Verification items for the finished model (mm, model axes). A direction names the side the tool comes from. Round coordinates to 2 decimals unless told otherwise and drop trailing zeros. Order: outer loops, then holes, each group sorted by start corner. A loop starts at its lowest first (then second) coordinate and runs counter-clockwise, first axis right, second up. Notation, with made-up numbers: (5, 61) -> (46, 61) arc R9 cw to (46, 74) -> close; hole circle Ø4 at (59.5, -17). An arc over 180 degrees is marked (long way). Return JSON: item names as keys, results as strings. Group by question number.
1) Tool access check on faces 4 (the flat face through (61.7, 2, 1)), 5 (the flat face through (20, 6.426, 1)), 6 (the flat face through (54.8, -17, 1)), 7 (the flat face through (61, 13.92, 1)). Record the directions out of +Z, -Z, +X, -X, +Y, -Y that give a thin tool (end or side, any length) a straight path to the whole face; none if there is none.
2) Section check C-C on y = 3. Enter the section's corners in (x, z), plus the area to 3 significant figures.
3) Scan lines: L1, parallel to Y at x = 63.3, z = 1.45; L2, parallel to Y at x = 19.5, z = 0.65; L3, parallel to X at y = 0, z = 0.5. Record each from-to range of solid material in increasing order.
4) Depth check by flat-ended pin: pin 1 (1.5 mm diameter, centred on x = 61.5, z = 1.5, fed in from -Y); pin 2 (1.5 mm diameter, centred on y = 2, z = 1, fed in from -X); pin 3 (1.6 mm diameter, centred on x = 15.5, z = 1.5, fed in from -Y); pin 4 (12 mm diameter, centred on x = 59, y = -8.5, fed in from -Z). Enter the tip coordinate at first touch or a pass-through.
5) Section check A-A on x = 19.5. Enter the section's corners in (y, z).
6) Draft check along Y on faces 1 (the flat face through (39.8, -17, 1)), 2 (the flat face through (31, -15.18, 1)), 3 (the flat face through (38.14, 2.58, 1.48)). Enter one of: pulls with the +Y half, pulls with the -Y half, needs draft (parallel to the pull), parting line crosses it, or undercut.
7) Section check B-B on x = 62.5. Enter the section's corners in (y, z).
8) Section check D-D on z = 1.65. State how many separate pieces and enclosed holes the cut face has, plus the area to 3 significant figures.
```python
from build123d import *

# Parameters (mm, degrees)
SKETCH_1_R           = 1.8
SKETCH_1_W           = 3
SKETCH_1_H           = 12
EXTRUDE_1_DEPTH      = 3
SKETCH_3_W           = 34
SKETCH_3_H           = 3
CUT_EXTRUDE_1_DEPTH  = 10
SKETCH_4_W           = 38
SKETCH_4_H           = 2
CUT_EXTRUDE_2_DEPTH  = 10
SKETCH_5_W           = 3
SKETCH_5_H           = 2
EXTRUDE_2_DEPTH      = 2
SKETCH_6_W           = 3
SKETCH_6_H           = 2
EXTRUDE_3_DEPTH      = 2
SKETCH_7_W           = 34
SKETCH_7_H           = 3
CUT_EXTRUDE_3_DEPTH  = 2
SKETCH_8_W           = 3
SKETCH_8_H           = 10
EXTRUDE_4_DEPTH      = 5
SKETCH_9_W           = 5
SKETCH_9_H           = 3
CUT_EXTRUDE_4_DEPTH  = 2
CUT_EXTRUDE_5_DEPTH  = 10
SKETCH_11_W          = 3
SKETCH_11_H          = 8
CUT_EXTRUDE_6_DEPTH  = 5
SKETCH_12_W          = 3.2
SKETCH_12_H          = 12.2
SKETCH_12_W_2        = 3
SKETCH_12_H_2        = 12
CUT_EXTRUDE_7_DEPTH  = 10
SKETCH_13_W          = 3.2
SKETCH_13_H          = 3
EXTRUDE_5_DEPTH      = 3
SKETCH_14_W          = 3.2
SKETCH_14_H          = 3
CUT_EXTRUDE_8_DEPTH  = 3
SKETCH_15_W          = 3.2
SKETCH_15_H          = 3
EXTRUDE_6_DEPTH      = 1
SKETCH_16_R          = 1.4
CUT_EXTRUDE_9_DEPTH  = 3
SKETCH_17_W          = 5
SKETCH_17_H          = 3.106186253
CUT_EXTRUDE_10_DEPTH = 10


with BuildPart() as part:
    # 草图1 → 凸台-拉伸1 (new body)
    with BuildSketch(Plane.XY):
        Polygon((-64.8, 13.92), (-67.8, 13.92), (-70.8, 10.92), (-70.8, -12.18), (-67.8, -15.18), (-64.8, -15.18), (-54.8, -15.18), (-54.8, -17.98), (-39.8, -17.98), (-39.8, -15.18), (-22, -15.18), (-22, 3.32), (-17, 3.32), (-17, 0.32), (17, 0.32), (17, 3.32), (22, 3.32), (22, -15.18), (39.8, -15.18), (39.8, -17.98), (54.8, -17.98), (54.8, -15.18), (67.8, -15.18), (70.8, -12.18), (70.8, 10.92), (67.8, 13.92), (54.8, 13.92), (54.8, 16.72), (29.8, 16.72), (29.8, 13.92), (10, 13.92), (10, 16.72), (-10, 16.72), (-10, 13.92), (-29.8, 13.92), (-29.8, 16.72), (-54.8, 16.72), (-54.8, 13.92), align=None)
        with Locations((-19.5, 10.636938849)):
            Circle(SKETCH_1_R, mode=Mode.SUBTRACT)
        with Locations((19.5, 10.636938849)):
            Circle(SKETCH_1_R, mode=Mode.SUBTRACT)
        with BuildLine():
            Line((-48.112743691, -4.863700543), (-43.239089288, 0.009953861))
            ThreePointArc((-43.239089288, 0.009953861), (-43.026957254, 0.097821826), (-42.814825219, 0.009953861))
            Line((-42.814825219, 0.009953861), (-40.739089288, -2.065782071))
            ThreePointArc((-40.739089288, -2.065782071), (-40.651221322, -2.277914105), (-40.739089288, -2.490046139))
            Line((-40.739089288, -2.490046139), (-43.380510644, -5.131467496))
            ThreePointArc((-43.380510644, -5.131467496), (-44.029357342, -5.565012998), (-44.794724207, -5.717253933))
            Line((-44.794724207, -5.717253933), (-47.759190301, -5.717253933))
            ThreePointArc((-47.759190301, -5.717253933), (-48.221130067, -5.408595649), (-48.112743691, -4.863700543))
        make_face(mode=Mode.SUBTRACT)
        with Locations((-63.3, -0.08)):
            Rectangle(SKETCH_1_W, SKETCH_1_H, mode=Mode.SUBTRACT)
        with BuildLine():
            Line((-37.309442832, -3.374108183), (-45.06249116, 4.378940145))
            ThreePointArc((-45.06249116, 4.378940145), (-45.170877535, 4.923835251), (-44.708937769, 5.232493535))
            Line((-44.708937769, 5.232493535), (-43.744471675, 5.232493535))
            ThreePointArc((-43.744471675, 5.232493535), (-42.97910481, 5.0802526), (-42.330258113, 4.646707097))
            Line((-42.330258113, 4.646707097), (-34.577209785, -3.10634123))
            ThreePointArc((-34.577209785, -3.10634123), (-34.46882341, -3.651236336), (-34.930763176, -3.95989462))
            Line((-34.930763176, -3.95989462), (-35.89522927, -3.95989462))
            ThreePointArc((-35.89522927, -3.95989462), (-36.660596135, -3.807653685), (-37.309442832, -3.374108183))
        make_face(mode=Mode.SUBTRACT)
        with BuildLine():
            Line((-32.819850472, 5.429192676), (-36.693504876, 1.555538273))
            ThreePointArc((-36.693504876, 1.555538273), (-36.90563691, 1.467670307), (-37.117768944, 1.555538273))
            Line((-37.117768944, 1.555538273), (-39.193504876, 3.631274204))
            ThreePointArc((-39.193504876, 3.631274204), (-39.281372841, 3.843406239), (-39.193504876, 4.055538273))
            Line((-39.193504876, 4.055538273), (-37.55208352, 5.696959629))
            ThreePointArc((-37.55208352, 5.696959629), (-36.903236822, 6.130505132), (-36.137869957, 6.282746067))
            Line((-36.137869957, 6.282746067), (-33.173403863, 6.282746067))
            ThreePointArc((-33.173403863, 6.282746067), (-32.711464097, 5.974087783), (-32.819850472, 5.429192676))
        make_face(mode=Mode.SUBTRACT)
        with Locations((63.3, -0.076886306)):
            Rectangle(SKETCH_1_W, SKETCH_1_H, mode=Mode.SUBTRACT)
        with BuildLine():
            Line((42.330258113, 4.646707097), (34.577209785, -3.10634123))
            ThreePointArc((34.577209785, -3.10634123), (34.46882341, -3.651236336), (34.930763176, -3.95989462))
            Line((34.930763176, -3.95989462), (35.89522927, -3.95989462))
            ThreePointArc((35.89522927, -3.95989462), (36.660596135, -3.807653685), (37.309442832, -3.374108183))
            Line((37.309442832, -3.374108183), (45.06249116, 4.378940145))
            ThreePointArc((45.06249116, 4.378940145), (45.170877535, 4.923835251), (44.708937769, 5.232493535))
            Line((44.708937769, 5.232493535), (43.744471675, 5.232493535))
            ThreePointArc((43.744471675, 5.232493535), (42.97910481, 5.0802526), (42.330258113, 4.646707097))
        make_face(mode=Mode.SUBTRACT)
        with BuildLine():
            Line((48.112743691, -4.863700543), (43.239089288, 0.009953861))
            ThreePointArc((43.239089288, 0.009953861), (43.026957254, 0.097821826), (42.814825219, 0.009953861))
            Line((42.814825219, 0.009953861), (40.739089288, -2.065782071))
            ThreePointArc((40.739089288, -2.065782071), (40.651221322, -2.277914105), (40.739089288, -2.490046139))
            Line((40.739089288, -2.490046139), (43.380510644, -5.131467496))
            ThreePointArc((43.380510644, -5.131467496), (44.029357342, -5.565012998), (44.794724207, -5.717253933))
            Line((44.794724207, -5.717253933), (47.759190301, -5.717253933))
            ThreePointArc((47.759190301, -5.717253933), (48.221130067, -5.408595649), (48.112743691, -4.863700543))
        make_face(mode=Mode.SUBTRACT)
        with BuildLine():
            Line((39.193504876, 4.055538273), (37.55208352, 5.696959629))
            ThreePointArc((37.55208352, 5.696959629), (36.903236822, 6.130505132), (36.137869957, 6.282746067))
            Line((36.137869957, 6.282746067), (33.173403863, 6.282746067))
            ThreePointArc((33.173403863, 6.282746067), (32.711464097, 5.974087783), (32.819850472, 5.429192676))
            Line((32.819850472, 5.429192676), (36.693504876, 1.555538273))
            ThreePointArc((36.693504876, 1.555538273), (36.90563691, 1.467670307), (37.117768944, 1.555538273))
            Line((37.117768944, 1.555538273), (39.193504876, 3.631274204))
            ThreePointArc((39.193504876, 3.631274204), (39.281372841, 3.843406239), (39.193504876, 4.055538273))
        make_face(mode=Mode.SUBTRACT)
    extrude(amount=EXTRUDE_1_DEPTH)

    # 草图3 → 切除-拉伸1 (cut)
    with BuildSketch(Plane(origin=(0, 0, 0), x_dir=(-1, 0, 0), z_dir=(0, 0, -1))):
        with Locations((0, 1.82)):
            Rectangle(SKETCH_3_W, SKETCH_3_H)
    extrude(amount=-CUT_EXTRUDE_1_DEPTH, mode=Mode.SUBTRACT)

    # 草图4 → 切除-拉伸2 (cut)
    with BuildSketch(Plane(origin=(0, 0, 0), x_dir=(-1, 0, 0), z_dir=(0, 0, -1))):
        with Locations((0, 4.32)):
            Rectangle(SKETCH_4_W, SKETCH_4_H)
    extrude(amount=-CUT_EXTRUDE_2_DEPTH, mode=Mode.SUBTRACT)

    # 草图5 → 凸台-拉伸2 (add)
    with BuildSketch(Plane(origin=(-19, 0, 0), x_dir=(0, 0, -1), z_dir=(1, 0, 0))):
        with Locations((-1.5, 4.32)):
            Rectangle(SKETCH_5_W, SKETCH_5_H)
    extrude(amount=EXTRUDE_2_DEPTH)

    # 草图6 → 凸台-拉伸3 (add)
    with BuildSketch(Plane.ZY.offset(-19)):
        with Locations((1.5, 4.32)):
            Rectangle(SKETCH_6_W, SKETCH_6_H)
    extrude(amount=EXTRUDE_3_DEPTH)

    # 草图7 → 切除-拉伸3 (cut)
    with BuildSketch(Plane.XZ.offset(-5.32)):
        with Locations((0, 1.5)):
            Rectangle(SKETCH_7_W, SKETCH_7_H)
    extrude(amount=-CUT_EXTRUDE_3_DEPTH, mode=Mode.SUBTRACT)

    # 草图8 → 凸台-拉伸4 (add)
    with BuildSketch(Plane.ZY.offset(-22)):
        with Locations((1.5, -7.18)):
            Rectangle(SKETCH_8_W, SKETCH_8_H)
    extrude_4 = extrude(amount=EXTRUDE_4_DEPTH)

    # 镜向1: 凸台-拉伸4 across plane
    add(extrude_4.mirror(Plane.ZY))

    # 草图9 → 切除-拉伸4 (cut)
    with BuildSketch(Plane.XZ.offset(12.18)):
        with Locations((-19.5, 1.5)):
            Rectangle(SKETCH_9_W, SKETCH_9_H)
        with Locations((19.5, 1.5)):
            Rectangle(SKETCH_9_W, SKETCH_9_H)
    extrude(amount=-CUT_EXTRUDE_4_DEPTH, mode=Mode.SUBTRACT)

    # 草图10 → 切除-拉伸5 (cut)
    with BuildSketch(Plane(origin=(0, 0, 0), x_dir=(-1, 0, 0), z_dir=(0, 0, -1))):
        Polygon((-15, 7.32), (-15, 18.727392341), (81.723481171, 18.727392341), (81.723481171, -24.797051458), (-15, -24.797051458), align=None)
    extrude(amount=-CUT_EXTRUDE_5_DEPTH, mode=Mode.SUBTRACT)

    # 草图11 → 切除-拉伸6 (cut)
    with BuildSketch(Plane.ZY.offset(-17)):
        with Locations((1.5, -6.18)):
            Rectangle(SKETCH_11_W, SKETCH_11_H)
    extrude(amount=-CUT_EXTRUDE_6_DEPTH, mode=Mode.SUBTRACT)

    # 草图12 → 切除-拉伸7 (cut)
    with BuildSketch(Plane(origin=(0, 0, 0), x_dir=(-1, 0, 0), z_dir=(0, 0, -1))):
        with Locations((-63.3, -0.076886306)):
            Rectangle(SKETCH_12_W, SKETCH_12_H)
        with Locations((-63.3, -0.076886306)):
            Rectangle(SKETCH_12_W_2, SKETCH_12_H_2, mode=Mode.SUBTRACT)
    extrude(amount=-CUT_EXTRUDE_7_DEPTH, mode=Mode.SUBTRACT)

    # 草图13 → 凸台-拉伸5 (add)
    with BuildSketch(Plane(origin=(0, -6.176886306, 0), x_dir=(1, 0, 0), z_dir=(0, 1, 0))):
        with Locations((63.3, -1.5)):
            Rectangle(SKETCH_13_W, SKETCH_13_H)
    extrude(amount=EXTRUDE_5_DEPTH)

    # 草图14 → 切除-拉伸8 (cut)
    with BuildSketch(Plane.XZ.offset(-6.023113694)):
        with Locations((63.3, 1.5)):
            Rectangle(SKETCH_14_W, SKETCH_14_H)
    extrude(amount=-CUT_EXTRUDE_8_DEPTH, mode=Mode.SUBTRACT)

    # 草图15 → 凸台-拉伸6 (add)
    with BuildSketch(Plane.XZ.offset(-9.023113694)):
        with Locations((63.3, 1.5)):
            Rectangle(SKETCH_15_W, SKETCH_15_H)
    extrude(amount=EXTRUDE_6_DEPTH)

    # 草图16 → 切除-拉伸9 (cut)
    with BuildSketch(Plane(origin=(-133.943153128, 43.327317851, 0), x_dir=(-1, 0, 0), z_dir=(0, 0, -1))):
        with Locations((-197.243153128, -51.882049417)):
            Circle(SKETCH_16_R)
    extrude(amount=-CUT_EXTRUDE_9_DEPTH, mode=Mode.SUBTRACT)

    # 草图17 → 切除-拉伸10 (cut)
    with BuildSketch(Plane(origin=(-133.943153128, 43.327317851, 0), x_dir=(-1, 0, 0), z_dir=(0, 0, -1))):
        with Locations((-153.443153128, -38.454224725)):
            Rectangle(SKETCH_17_W, SKETCH_17_H)
    extrude(amount=-CUT_EXTRUDE_10_DEPTH, mode=Mode.SUBTRACT)


solid = part.part
```
Check result:
{
 "1": {"face 4": "+Z, -Z", "face 5": "+Z, -Z, -X, -Y", "face 6": "+Z, -Z, +X, -Y", "face 7": "+Z, -Z, +X, +Y"},
 "2": {"outline": "(22, 0) -> (35.25, 0) -> (35.25, 3) -> (22, 3) -> close; (38.56, 0) -> (40.68, 0) -> (40.68, 3) -> (38.56, 3) -> close; (43.68, 0) -> (61.7, 0) -> (61.7, 3) -> (43.68, 3) -> close; (64.9, 0) -> (70.8, 0) -> (70.8, 3) -> (64.9, 3) -> close", "area": "118 mm^2"},
 "3": {"L1": "-15.18 to -9.95, -7.15 to -3.18, 8.02 to 13.92", "L2": "6.43 to 8.84, 12.44 to 13.92", "L3": "22 to 37.68, 40.68 to 42.8, 43.25 to 61.7, 64.9 to 70.8"},
 "4": {"pin 1": "y = -15.18", "pin 2": "x = 22", "pin 3": "y = 7.32", "pin 4": "z = 0"},
 "5": {"outline": "(6.43, 0) -> (8.84, 0) -> (8.84, 3) -> (6.43, 3) -> close; (12.44, 0) -> (13.92, 0) -> (13.92, 3) -> (12.44, 3) -> close"},
 "6": {"face 1": "needs draft", "face 2": "pulls with the -Y half", "face 3": "undercut"},
 "7": {"outline": "(-15.18, 0) -> (-9.7, 0) -> (-9.7, 3) -> (-15.18, 3) -> close; (-7.41, 0) -> (-3.18, 0) -> (-3.18, 3) -> (-7.41, 3) -> close; (8.02, 0) -> (13.92, 0) -> (13.92, 3) -> (8.02, 3) -> close"},
 "8": {"separate pieces": "1", "enclosed holes": "6", "area": "1,450 mm^2"}
}
